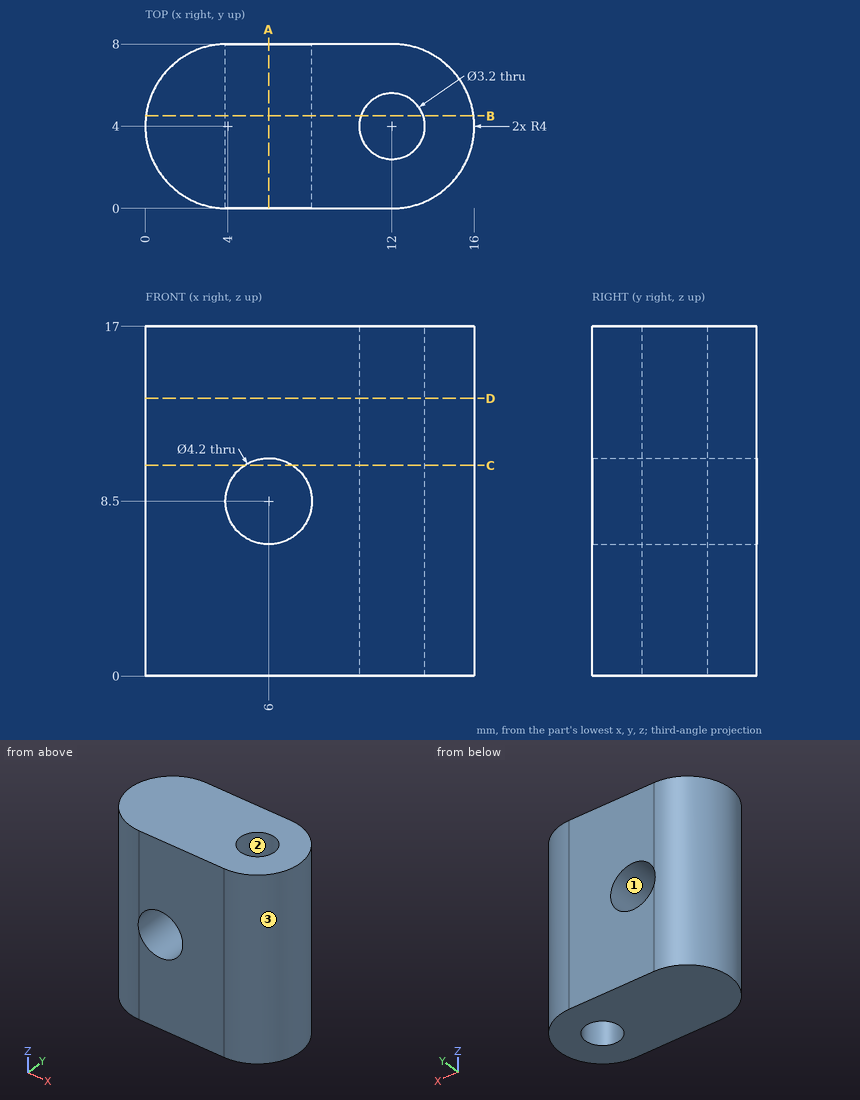
Input: dimensioned drawing with shaded views. Units: mm. Origin: part minimum x, y, z. Round coordinates to 2 decimals unless told otherwise and drop trailing zeros. Order: outer loops, then holes, each group sorted by start corner. A loop starts at its lowest first (then second) coordinate and runs counter-clockwise, first axis right, second up.
Q1. Material intervals for probe 1 along Z at (x, y) = (6, 2); probe 2 along X at (y, z) = (5.25, 7.75); probe 3 along X at (y, z) = (3, 8.25), sorted ascending.
Result sheet:
probe 1: z = 0 to 6.4, 10.6 to 17
probe 2: x = 0.2 to 4.04, 7.96 to 11, 13 to 15.8
probe 3: x = 0.13 to 3.91, 8.09 to 10.75, 13.25 to 15.87
Q2. Section B-B, the plane y = 4.5. Output: boundary loops of the cut face in (x, z).
Result sheet:
outline: (0.03, 0) - (10.48, 0) - (10.48, 17) - (0.03, 17) - close; (13.52, 0) - (15.97, 0) - (15.97, 17) - (13.52, 17) - close; hole circle Ø4.2 at (6, 8.5)
Q3. Mould query, pull axis Y, two halves, no side actions, for the marked faces 1, 2 and 3. Classes: released by +Y, released by -Y, zero draft, split by the parting line, or undercut.
Result sheet:
face 1: zero draft
face 2: undercut
face 3: split by the parting line
Q4. Section A-A, the plane x = 6. Output: boundary loops of the cut face in (y, z), and give its area (3 significant figures).
Result sheet:
outline: (0, 0) - (8, 0) - (8, 6.4) - (0, 6.4) - close; (0, 10.6) - (8, 10.6) - (8, 17) - (0, 17) - close
area: 102 mm2
Q5. Pin query (flat end, axial travel): pin 1 (3 mm diameter, centred on y = 7, z = 4.5, fed in from -X); pin 2 (1.5 mm diameter, centred on x = 12.5, y = 3, fed in from +Z); pin 3 (2 mm diameter, centred on y = 7, z = 8.5, fed in from -X). Return the tip coordinate at first contact, or that it passes through.
Result sheet:
pin 1: stops at x = 0.29
pin 2: stops at z = 17
pin 3: stops at x = 0.54
Q6. Section C-C, the plane z = 10.25. Output: boundary loops of the cut face in (x, y).
Result sheet:
outline: (4, 0) - (4.84, 0) - (4.84, 8) - (4, 8) arc R4 ccw to start; (7.16, 0) - (12, 0) arc R4 ccw to (12, 8) - (7.16, 8) - close; hole circle Ø3.2 at (12, 4)
Q7. Section D-D, the plane z = 13.5. Output: boundary loops of the cut face in (x, y).
Result sheet:
outline: (4, 0) - (12, 0) arc R4 ccw to (12, 8) - (4, 8) arc R4 ccw to start; hole circle Ø3.2 at (12, 4)
